The model under review builds one solid part; all positions refer to its coordinate system, in mm. A direction names the side the tool comes from. Coordinates: 2 decimals unless noted, no trailing zeros. Write each loop counter-clockwise with the first axis right and the second up, starting at its lowest first coordinate (ties: lowest second). Pieces come first, ordered by that corner, then holes. Notation, with made-up numbers: M 52.5,53.5 L 108.5,53.5 A17 ccw 108.5,84.5 Z; hole C 12,78.25 d7. An arc over 180 degrees is marked long. Answer as a JSON object with one key per item and string values.
```python
from build123d import *

# Parameters (mm, degrees)
SKETCH1_W           = 75
SKETCH1_H           = 23
BOSS_EXTRUDE1_DEPTH = 3
BOSS_EXTRUDE4_DEPTH = 5
SKETCH3_W           = 10.5
SKETCH3_H           = 1
BOSS_EXTRUDE5_DEPTH = 48.5
SKETCH4_R           = 2
CUT_EXTRUDE1_DEPTH  = 66.282886378


with BuildPart() as part:
    # Sketch1 → Boss-Extrude1 (new body)
    with BuildSketch(Plane(origin=(0, 0, 0), x_dir=(1, 0, 0), z_dir=(0, 1, 0))):
        Rectangle(SKETCH1_W, SKETCH1_H)
    extrude(amount=BOSS_EXTRUDE1_DEPTH)

    # Sketch2 → Boss-Extrude4 (add)
    with BuildSketch(Plane.XY.offset(11.5)):
        Polygon((27.230257431, 0), (27.230257431, -45.514890462), (26.230257431, -45.514890462), (26.230257431, 3), (36.730257431, 3), (36.730257431, -45.514890462), (35.730257431, -45.514890462), (35.730257431, 0), align=None)
        Polygon((-35.730257431, -45.514890462), (-36.730257431, -45.514890462), (-36.730257431, 3), (-26.230257431, 3), (-26.230257431, -45.514890462), (-27.230257431, -45.514890462), (-27.230257431, 0), (-35.730257431, 0), align=None)
    extrude(amount=BOSS_EXTRUDE4_DEPTH)

    # Sketch3 → Boss-Extrude5 (add)
    with BuildSketch(Plane.XZ.offset(45.514890462)):
        with Locations((-31.480257431, 17)):
            Rectangle(SKETCH3_W, SKETCH3_H)
        with Locations((31.480257431, 17)):
            Rectangle(SKETCH3_W, SKETCH3_H)
    extrude(amount=-BOSS_EXTRUDE5_DEPTH)

    # Sketch4 → Cut-Extrude1 (cut, through all)
    with BuildSketch(Plane(origin=(0, 0, 16.5), x_dir=(-1, 0, 0), z_dir=(0, 0, -1))):
        with Locations((31.481258109, -34.012149814)):
            Circle(SKETCH4_R)
        with Locations((-31.503449984, -34.014890462)):
            Circle(SKETCH4_R)
    extrude(amount=-CUT_EXTRUDE1_DEPTH, mode=Mode.SUBTRACT)


solid = part.part
```
(1) Wall thickness on line 1 along X through (y, z) = (-7, 12.25); line 2 along Y through (x, z) = (32, -3); line 3 along Z through (x, y) = (-29, -18): over which ranges is each line inside the solid? List them lowest first. Write a range as from..to.
Results list:
{"line 1": "-36.73..-35.73, -27.23..-26.23, 26.23..27.23, 35.73..36.73", "line 2": "0..3", "line 3": "16.5..17.5"}
(2) For pin 1 Ø3 at (y, z) = (-13, 14) entering from +X; pin 2 Ø5 at (x, z) = (-22, -4) entering from -Y; pin 3 Ø0.8 at (x, z) = (29, 17) entering from +Y, all flat-tipped, find the tip position at first contact; note any pin that passes through.
Results list:
{"pin 1": "x = 36.73", "pin 2": "y = 0", "pin 3": "y = 2.99"}
(3) For faces 1 (the face through (0, 1, 11.5)), 2 (the face through (-32, -45.515, 17)), 3 (the face through (-32, -23, 16.5)), list the 3-axis set-ups (+Z, -Z, +X, -X, +Y, -Y) from which the entire face can be reached by the end or side of a thin tool; tool diameter is ignored.
Results list:
{"face 1": "+Z, +Y, -Y", "face 2": "+Z, -Z, +X, -X, -Y", "face 3": "-Z, -Y"}
(4) Add section A-A on y = -38. Give the boundary of the cut face in (x, z).
Results list:
{"outline": "M -36.73,11.5 L -35.73,11.5 L -35.73,16.5 L -27.23,16.5 L -27.23,11.5 L -26.23,11.5 L -26.23,17.5 L -36.73,17.5 Z; M 26.23,11.5 L 27.23,11.5 L 27.23,16.5 L 35.73,16.5 L 35.73,11.5 L 36.73,11.5 L 36.73,17.5 L 26.23,17.5 Z"}
(5) Draft analysis for pull direction X (two halves, no side actions). For faces 4 (the face through (36.73, -21, 14)), 5 (the face through (-37.5, 1, 0)), 6 (the face through (31, -23, 16.5)), state which applies: released by +X, released by -X, zero draft, split by the parting line, or undercut.
Results list:
{"face 4": "released by +X", "face 5": "released by -X", "face 6": "undercut"}
(6) Add section D-D on x = 24. Give the boundary of the cut face in (y, z), and give its area (3 significant figures).
Results list:
{"outline": "M 0,-11.5 L 3,-11.5 L 3,11.5 L 0,11.5 Z", "area": "69.0 mm²"}
(7) Add section B-B on z = 14.5. Give the boundary of the cut face in (x, y).
Results list:
{"outline": "M -36.73,-45.51 L -35.73,-45.51 L -35.73,0 L -27.23,0 L -27.23,-45.51 L -26.23,-45.51 L -26.23,3 L -36.73,3 Z; M 26.23,-45.51 L 27.23,-45.51 L 27.23,0 L 35.73,0 L 35.73,-45.51 L 36.73,-45.51 L 36.73,3 L 26.23,3 Z"}
